```python
from build123d import *

# Parameters (mm, degrees)
FILLET_1_R = 1
SHELL_1_T  = -1


with BuildPart() as part:
    # Эскиз1 → Повернуть1 (revolve)
    with BuildSketch(Plane.XY):
        Polygon((0, 0), (-10, 0), (-10, 20), (-16, 26), (-16, 33), (0, 33), align=None)
    revolve(axis=Axis((0, 33, 0), (0, -1, 0)))

    # Скругление1
    fillet_1_edges = [part.edges().sort_by_distance(p)[0] for p in [
        (16, 26, 0),
        (10, 20, 0),
    ]]
    fillet(fillet_1_edges, radius=FILLET_1_R)

    # Оболочка1
    shell_1_openings = [part.faces().sort_by_distance(p)[0] for p in [
        (0, 33, 0),
        (0, 0, 0),
    ]]
    offset(amount=SHELL_1_T, openings=shell_1_openings, kind=Kind.INTERSECTION)


solid = part.part
```
Verification items for the finished model (mm, model axes). A direction names the side the tool comes from. Coordinates: 2 decimals unless noted, no trailing zeros. Loops run counter-clockwise (first coordinate to the right, second up) from the corner with the lowest first, then second, coordinate; pieces in that order, holes last. Notation, with made-up numbers: (-31, 37) - (-14, 37) arc R23 cw to (-14, 50) - close; hole circle Ø10 at (-29.5, -26.5). An arc over 180 degrees is marked (long way). Return JSON: item names as keys, results as strings.
1. Thickness scan on L1, parallel to X at y = 28.25, z = 0; L2, parallel to Z at x = 0, y = 5.5. Record the ranges inside material, lowest first.
Established:
{"L1": "x = -16 to -15, 15 to 16", "L2": "z = -10 to -9, 9 to 10"}
2. Mould release check, pull along X, two halves, no side actions. Record for faces 3 (the flat face through (-9, 0, -2)), 4 (the conical face through (-10.14, 20.63, -3.19)), 5 (the cylindrical face through (-13.856, 29.753, 5.745)): +X half, -X half, draft (parallel to the pull), parting line (faces both ways), or undercut.
Established:
{"face 3": "draft", "face 4": "parting line", "face 5": "undercut"}
3. Tool access check on faces 1 (the conical face through (-9.47, 21.34, -2.98)), 2 (the cylindrical face through (-5.38, 9.93, -8.43)). Record the directions out of +Z, -Z, +X, -X, +Y, -Y that give a thin tool (end or side, any length) a straight path to the whole face; none if there is none.
Established:
{"face 1": "+Y", "face 2": "-Y"}
4. Section check C-C, the plane y = 28.5. Record the boundary of the cut face in (x, z), then the cut area to 3 significant figures.
Established:
{"outline": "circle Ø32 at (0, 0); hole circle Ø30 at (0, 0)", "area": "97.4 mm2"}
5. Go/stop test with flat-tipped pins: pin 1 (8 mm diameter, centred on y = 7.5, z = 6, fed in from +X); pin 2 (5 mm diameter, centred on y = 6.5, z = 7, fed in from +X); pin 3 (5 mm diameter, centred on x = 5, y = 22, fed in from +Z). Record where each tip stops, or that it passes through.
Established:
{"pin 1": "stops at x = 9.8", "pin 2": "stops at x = 8.93", "pin 3": "stops at z = 13.74"}
6. Section check A-A, the plane y = 10.5. Record the boundary of the cut face in (x, z).
Established:
{"outline": "circle Ø20 at (0, 0); hole circle Ø18 at (0, 0)"}
